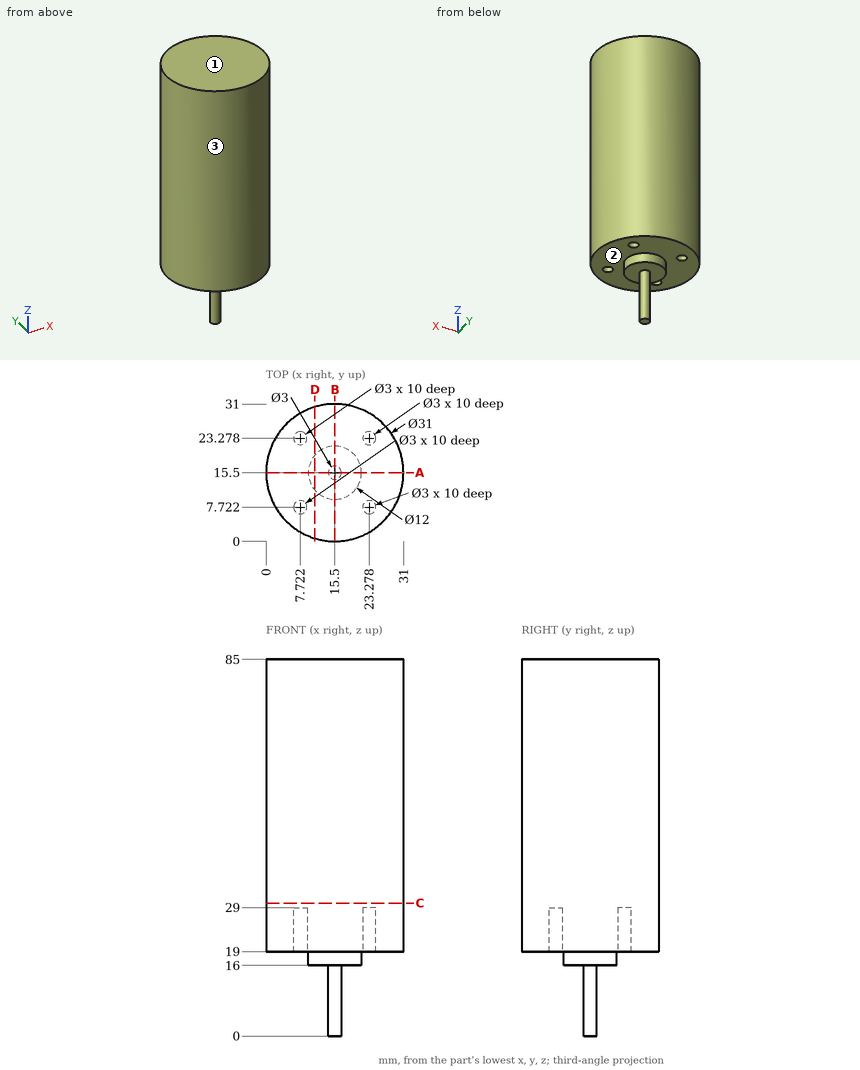
Verification items for this drawing (mm, ordinates from the low corner). Coordinates: 2 decimals unless noted, no trailing zeros. Write each loop counter-clockwise with the first axis right and the second up, starting at its lowest first coordinate (ties: lowest second). Pieces come first, ordered by that corner, then holes. Notation, with made-up numbers: M 26.5,35 L 48.5,35 A19 cw 48.5,68 Z; hole C -37,30.25 d6. An arc over 180 degrees is marked long. Use one line per item in the form item = value. Start each with the question number.
1) Go/stop test with flat-tipped pins: pin 1 Ø5 at (x, z) = (6.5, 55) entering from -Y; pin 2 Ø3.5 at (x, y) = (8.5, 8.5) entering from -Z; pin 3 Ø12 at (x, z) = (7.5, 20.5) entering from +Y. Record where each tip stops, or that it passes through.
2) Thickness scan on probe 1 along Y at (x, z) = (15.5, 58); probe 2 along Z at (x, y) = (9, 18); probe 3 along Y at (x, z) = (15.5, 15). Record the ranges inside material, lowest first. Write a range as from..to.
3) Section check C-C on z = 30. Enter the section's corners in (x, y), and give its area (3 significant figures).
4) Section check D-D on x = 11. Enter the section's corners in (y, z).
5) Section check A-A on y = 15.5. Enter the section's corners in (x, z).
6) Release check for a two-part mould opening along Z. For the marked faces 1, 2 and 3 record: pulls with the +Z half, pulls with the -Z half, needs draft (parallel to the pull), parting line crosses it, or undercut.
Responses:
q1.pin_1 = 1.43
q1.pin_2 = 19
q1.pin_3 = 30.87
q2.probe_1 = 0..31
q2.probe_2 = 19..85
q2.probe_3 = 14..17
q3.outline = C 15.5,15.5 d31
q3.area = 755 mm2
q4.outline = M 0.67,19 L 11.53,19 L 11.53,16 L 19.47,16 L 19.47,19 L 30.33,19 L 30.33,85 L 0.67,85 Z
q5.outline = M 0,19 L 9.5,19 L 9.5,16 L 14,16 L 14,0 L 17,0 L 17,16 L 21.5,16 L 21.5,19 L 31,19 L 31,85 L 0,85 Z
q6.face_1 = pulls with the +Z half
q6.face_2 = pulls with the -Z half
q6.face_3 = needs draft
